Input: dimensioned drawing with shaded views. Units: mm. Origin: part minimum x, y, z. A direction names the side the tool comes from. Round coordinates to 2 decimals unless told otherwise and drop trailing zeros. Loops run counter-clockwise (first coordinate to the right, second up) from the corner with the lowest first, then second, coordinate; pieces in that order, holes last. Notation, with made-up numbers: M 19.25,87.5 L 24.25,87.5 A22 cw 24.25,117.5 Z; hole C -4,-4.75 d2. An arc over 180 degrees is marked long. Put each result on its own line as item: value. Start each with the question number.
1) Reachability of the marked faces 4 and 5 from +Z, -Z, +X, -X, +Y, -Y: full face, straight path, thin tool, end or side. Return the list, or none.
2) Section B-B on x = 59. Output: boundary loops of the cut face in (y, z).
3) Pin query (flat end, axial travel): pin 1 (12.5 mm diameter, centred on y = 8, z = 89, fed in from -X). Return the tip coordinate at first contact, or that it passes through.
4) Draft query along Y for the marked faces 1, 2 and 3. Return one class per face: +Y half, -Y half, draft (parallel to the pull), parting line (faces both ways), or undercut.
5) Section A-A on y = 17.5. Output: boundary loops of the cut face in (x, z), plus the area to 3 significant figures.
6) Line query: probe 1 along X at (y, z) = (6.5, 88); probe 2 along Z at (x, y) = (17, 16); probe 3 along Y at (x, z) = (70.5, 101). Output: solid intervals per line, ascending.
7) Section C-C on z = 147.5. Output: boundary loops of the cut face in (x, y).
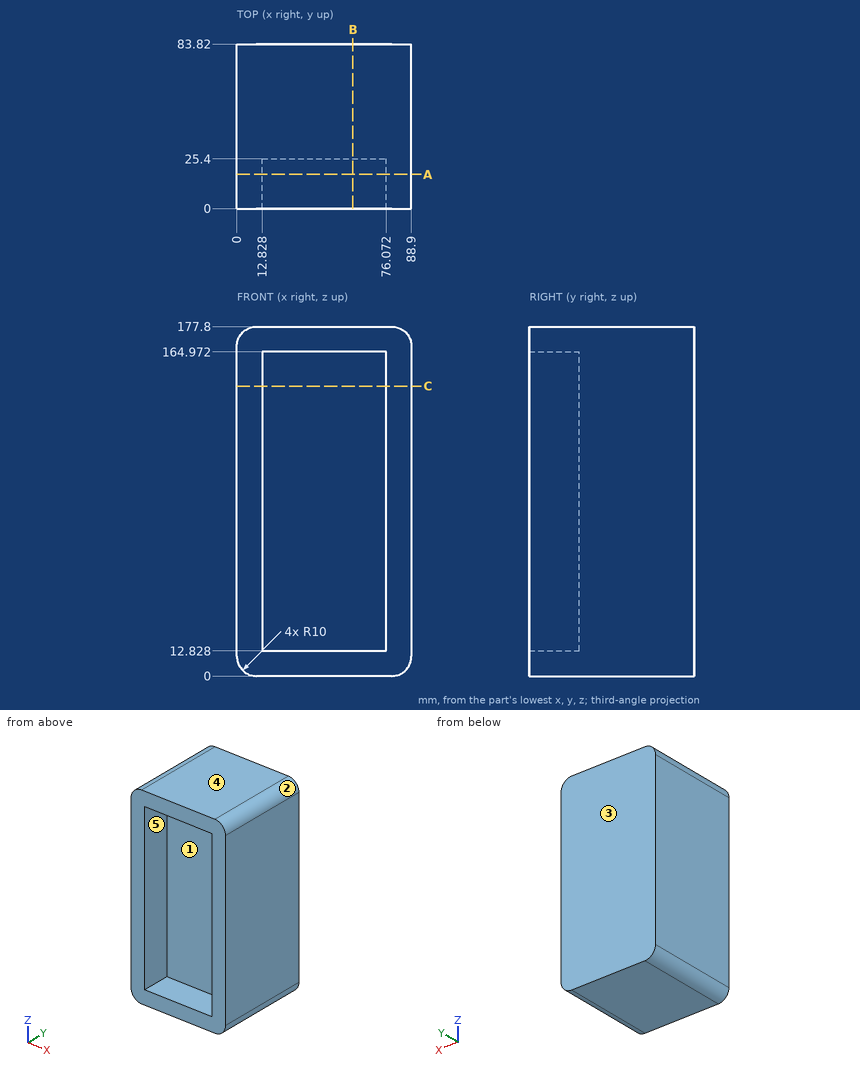
Geometry results:
1. face 4: +Z, +X, -X, +Y, -Y
1. face 5: -Y
2. outline: M 0,0 L 83.82,0 L 83.82,177.8 L 0,177.8 L 0,164.97 L 25.4,164.97 L 25.4,12.83 L 0,12.83 Z
3. pin 1: stops at x = 0
4. face 1: -Y half
4. face 2: draft
4. face 3: +Y half
5. outline: M 0,10 A10 ccw 10,0 L 78.9,0 A10 ccw 88.9,10 L 88.9,167.8 A10 ccw 78.9,177.8 L 10,177.8 A10 ccw 0,167.8 Z; hole M 12.83,12.83 L 76.07,12.83 L 76.07,164.97 L 12.83,164.97 Z
5. area: 6,100 mm²
6. probe 1: x = 0 to 12.83, 76.07 to 88.9
6. probe 2: z = 0 to 12.83, 164.97 to 177.8
6. probe 3: y = 25.4 to 83.82
7. outline: M 0,0 L 12.83,0 L 12.83,25.4 L 76.07,25.4 L 76.07,0 L 88.9,0 L 88.9,83.82 L 0,83.82 Z
